CAD build for the part. Positions are in the model's coordinates, mm. A direction names the side the tool comes from. Coordinates: 2 decimals unless noted, no trailing zeros. Order: outer loops, then holes, each group sorted by start corner. A loop starts at its lowest first (then second) coordinate and runs counter-clockwise, first axis right, second up. Notation, with made-up numbers: (6, 0) -> (10, 0) arc R23 cw to (10, 18) -> close; hole circle Ø5 at (-22.5, 50). An arc over 180 degrees is marked (long way). Use one line per item in the form item = value. Start each with the question number.
Autodesk Inventor part; units mm, degrees
ref_plane "YZ Plane" through (0, 0, 0) normal (1, 0, 0) x (0, 1, 0)
ref_plane "XZ Plane" through (0, 0, 0) normal (0, 1, 0) x (-1, 0, 0)
ref_plane "XY Plane" through (0, 0, 0) normal (0, 0, 1) x (1, 0, 0)
sketch "Szkic2" plane through (0, 0, 0) normal (1, 0, 0) x (0, 1, 0)
  line L0 (0, -2.9) -> (0, 2.9)
  line L1 (-1.5, -1.5) -> (-1.5, 1.5)
  line L2 (-1.5, -1.5) -> (0, -2.9)
  line L3 (-1.5, 1.5) -> (0, 2.9)
  line L4 (0, 0) -> (-20, 0)
  line L5 (-20, 0) -> (-20, -1.5)
  line L6 (-20, -1.5) -> (-1.5, -1.5)
  dimension "d0" = 5.8
  dimension "d2" = 3
  dimension "d3" = 1.5
  dimension "d4" = 20
  dimension "d5" = 1.5
revolve "Obrót1" add sketch "Szkic2" angle 360 about axis through (0, 0, 0) along (0, -1, 0) contours L2 L1 L4 L0 | L6 L5 L4 L1
sketch "Szkic3" plane through (0, 0, 0) normal (0, 1, 0) x (1, 0, 0)
  line L0 (-1.1673, -0.633) -> (-1.1318, 0.6945)
  line L1 (-1.1318, 0.6945) -> (0.0355, 1.3274)
  line L2 (0.0355, 1.3274) -> (1.1673, 0.633)
  line L3 (1.1673, 0.633) -> (1.1318, -0.6945)
  line L4 (1.1318, -0.6945) -> (-0.0355, -1.3274)
  line L5 (-0.0355, -1.3274) -> (-1.1673, -0.633)
  point P0 (0, 0)
  point P1 (0, 0)
  dimension "d7" = 2.3
extrude "Wyciągnięcie proste1" cut sketch "Szkic3" against normal blind 2
fillet "Zaokrąglenie1" radius 0.5 6 edges at (-1.1496, -2, -0.0308) (-0.6014, -2, 0.9802) (-0.5482, -2, -1.011) (0.6014, -2, -0.9802) (0.5482, -2, 1.011) (1.1496, -2, 0.0308)
fillet "Zaokrąglenie2" radius 0.5 1 edges at (0, -1.5, 1.5)
fillet "Zaokrąglenie3" radius 0.1 1 edges at (0, 0, 2.9)
thread "Gwint1"
chamfer "Faza1" distance 0.5 angle 45 1 edges at (0, -20, 1.5)
properties part number "Screw M3 20mm flat head"
1) Probe L1, parallel to Z at x = 0.7, y = -7.25; L2, parallel to Z at x = 1.3, y = -10. List the from-to ranges inside material, lowest first.
2) Two-plate mould, pull along Z, no slides. Class faces 1 (the face through (-0.593, -0.74, 0.985)), 2 (the face through (0.556, -0.74, 1.007)), 3 (the face through (-0.07, -10.47, 1.5)), 4 (the face through (-1, 0, -1)): released by +Z, released by -Z, zero draft, split by the parting line, or undercut.
3) Drop flat-ended pins along their axis: P1, Ø2, axis at x = 1, y = -4.5, coming from the -Z side; P2, Ø1.5, axis at x = 0, z = 0, coming from the +Y side; P3, Ø2, axis at x = 1.5, z = -1.5, coming from the -Y side. Give the stop position or say it passes through.
4) Cut at A-A on y = -17.25. Give the cut face in (x, z), then the cut area to 3 significant figures.
5) 3-axis set-ups, long thin cutter, end or side, ignore diameter. For faces 5 (the face through (0, -20, 0)), 6 (the face through (0, -2, 0)): which of +Z, -Z, +X, -X, +Y, -Y reach the whole face in a straight line?
Values follow:
q1.L1 = -1.33 to 1.33
q1.L2 = -0.75 to 0.75
q2.face_1 = undercut
q2.face_2 = undercut
q2.face_3 = split by the parting line
q2.face_4 = zero draft
q3.P1 = -1.5
q3.P2 = -1.99
q3.P3 = -19.88
q4.outline = circle Ø3 at (0, 0)
q4.area = 7.07 mm^2
q5.face_5 = +Z, -Z, +X, -X, -Y
q5.face_6 = +Y
